from build123d import *

# Parameters (mm, degrees)
F0_W     = 15
F0_H     = 130
F1_DEPTH = 60
F2_R     = 10
F3_DEPTH = 7.5
F4_R     = 10
F5_R     = 4.99999


# Not quite as in the source:
# - a fillet or chamfer is up to 0.001 mm smaller than in the source, because OpenCascade refuses the exact size


with BuildPart() as f1:
    # F0 (on Top) → F1 (new body)
    with BuildSketch(Plane.XY):
        Rectangle(F0_W, F0_H)
    extrude(amount=F1_DEPTH)

    # F2 (on face) → F3 (cut)
    with BuildSketch(Plane.YZ.offset(7.5)):
        with Locations((-50, 15)):
            Circle(F2_R)
        with Locations((50, 15)):
            Circle(F2_R)
    extrude(amount=-F3_DEPTH, mode=Mode.SUBTRACT)

    # F4
    f4_edges = [f1.edges().sort_by_distance(p)[0] for p in [
        (0, -65, 0),
        (0, 65, 0),
    ]]
    fillet(f4_edges, radius=F4_R)

    # F5 (radius 5 in the source; OpenCascade refuses exactly that, so slightly less here)
    f5_edges = [f1.edges().sort_by_distance(p)[0] for p in [
        (7.5, 0, 0),
        (-7.5, 0, 0),
    ]]
    fillet(f5_edges, radius=F5_R)


solid = f1.part
Build history of the part. All positions in model axes, mm. A direction names the side the tool comes from. Round coordinates to 2 decimals unless told otherwise and drop trailing zeros. Write each loop counter-clockwise with the first axis right and the second up, starting at its lowest first coordinate (ties: lowest second). Pieces come first, ordered by that corner, then holes. Notation, with made-up numbers: (17, 32) - (47, 32) arc R18 cw to (47, 59) - close; hole circle Ø2 at (15, 4). An arc over 180 degrees is marked (long way). One line per question, with ' | ' between items.
1. Drop a flat-ended pin along its axis: pin 1 Ø18 at (y, z) = (-50, 15) entering from +X. Give the stop position or say it passes through.
Results are:
pin 1: x = 0
2. Band-saw the part on C-C, the plane x = -5. Write the cut outline in (y, z), and give its area (3 significant figures).
Results are:
outline: (-64.33, 10) arc R9.33 ccw to (-55, 0.67) - (55, 0.67) arc R9.33 ccw to (64.33, 10) - (64.33, 60) - (-64.33, 60) - close | area: 7,600 mm^2
3. Mould opens along Z. For faces 3 (the face through (0, -65, 35)), 4 (the face through (6, 0.77, 1.43)), 5 (the face through (0, -50, 15)) say: released by +Z, released by -Z, zero draft, split by the parting line, or undercut.
Results are:
face 3: zero draft | face 4: released by -Z | face 5: undercut
4. Drill centre lines: line 1 along Z through (x, y) = (3, -50); line 2 along Z through (x, y) = (3.5, 50); line 3 along Z through (x, y) = (-2.75, 4). Where is each one in solid material? Low to high. Write a range as from..to.
Results are:
line 1: 0.03..5, 25..60 | line 2: 0.1..5, 25..60 | line 3: 0.01..60
5. Tool access for faces 1 (the face through (0, 50, 15)), 2 (the face through (7.5, -1, 32)): list every direction of +Z, -Z, +X, -X, +Y, -Y with a clear straight run to the whole face (end or side of a thin tool).
Results are:
face 1: +X | face 2: +Z, -Z, +X, +Y, -Y
